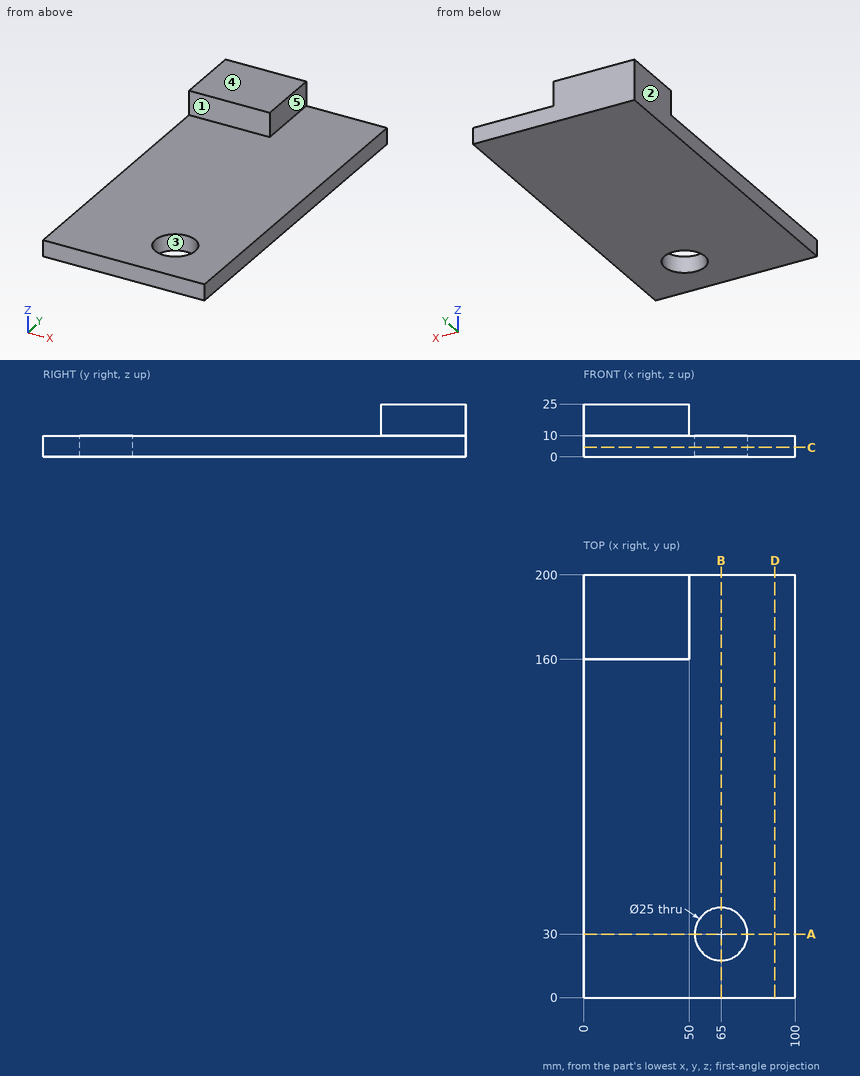
Drawing for the job (mm, zero at the part's lowest x, y, z). A direction names the side the tool comes from. Round coordinates to 2 decimals unless told otherwise and drop trailing zeros. Loops run counter-clockwise (first coordinate to the right, second up) from the corner with the lowest first, then second, coordinate; pieces in that order, holes last. Notation, with made-up numbers: (-36, -37.5) -> (-7, -37.5) arc R17 ccw to (-7, -30.5) -> close; hole circle Ø7 at (46, 74.5). An arc over 180 degrees is marked (long way). Use one line per item in the form item = value. Start each with the question number.
Item 1: Tool access for the marked faces 1 and 2: list every direction of +Z, -Z, +X, -X, +Y, -Y with a clear straight run to the whole face (end or side of a thin tool).
Item 2: Band-saw the part on D-D (x = 90.5). List the corners of the cut face in (y, z), plus the area to 3 significant figures.
Item 3: Band-saw the part on C-C (z = 4.5). List the corners of the cut face in (x, y).
Item 4: Two-plate mould, pull along X, no slides. Class the marked faces 3, 4 and 5: released by +X, released by -X, zero draft, split by the parting line, or undercut.
Item 5: Band-saw the part on A-A (y = 30). List the corners of the cut face in (x, z).
Item 6: Band-saw the part on B-B (x = 65). List the corners of the cut face in (y, z), plus the area to 3 significant figures.
Item 7: Drill centre lines: line 1 along Y through (x, z) = (65, 7.5); line 2 along Z through (x, y) = (86, 52); line 3 along Y through (x, z) = (36, 22). Where is each one in solid material? Low to high.
Item 8: Drop flat-ended pins along their axis: pin 1 Ø7.5 at (y, z) = (178.5, 16.5) entering from +X; pin 2 Ø6 at (x, y) = (26, 45.5) entering from +Z; pin 3 Ø12 at (x, z) = (27, 20) entering from -Y. Give the stop position or say it passes through.
Data:
q1.face_1 = +Z, +X, -X, -Y
q1.face_2 = +Z, -Z, -X, +Y, -Y
q2.outline = (0, 0) -> (200, 0) -> (200, 10) -> (0, 10) -> close
q2.area = 2,000 mm^2
q3.outline = (0, 0) -> (100, 0) -> (100, 200) -> (0, 200) -> close; hole circle Ø25 at (65, 30)
q4.face_3 = undercut
q4.face_4 = zero draft
q4.face_5 = released by +X
q5.outline = (0, 0) -> (52.5, 0) -> (52.5, 10) -> (0, 10) -> close; (77.5, 0) -> (100, 0) -> (100, 10) -> (77.5, 10) -> close
q6.outline = (0, 0) -> (17.5, 0) -> (17.5, 10) -> (0, 10) -> close; (42.5, 0) -> (200, 0) -> (200, 10) -> (42.5, 10) -> close
q6.area = 1,750 mm^2
q7.line_1 = 0 to 17.5, 42.5 to 200
q7.line_2 = 0 to 10
q7.line_3 = 160 to 200
q8.pin_1 = 50
q8.pin_2 = 10
q8.pin_3 = 160
